Job drawing, mm, ordinate dimensions from the low corner. One solid piece. Coordinates: 2 decimals unless noted, no trailing zeros. Write each loop counter-clockwise with the first axis right and the second up, starting at its lowest first coordinate (ties: lowest second). Pieces come first, ordered by that corner, then holes. Notation, with made-up numbers: (-33.5, 3) - (-29.5, 3) arc R16 cw to (-29.5, 9) - close; hole circle Ø7 at (73, 76). An arc over 180 degrees is marked (long way). Put each result on its own line as item: value. Start each with the question number.
1. Drill centre lines: L1, parallel to X at y = 312, z = 3.75; L2, parallel to Y at x = 27, z = 2 (3 decimals). Where is each one in solid material? Low to high. Write a range as from..to.
2. Saw through at A-A, the plane z = 1.75. Write the cut outline in (x, y) (3 decimals), plus the area to 3 significant figures.
3. Drop flat-ended pins along their axis: P1, Ø3, axis at y = 66, z = 2.5, coming from the +X side; P2, Ø3, axis at y = 57, z = 4, coming from the -X side; P3, Ø3, axis at x = 395.5, z = 4.5, coming from the -Y side (3 decimals). Give the stop position or say it passes through.
4. Saw through at C-C, the plane y = 71. Write the cut outline in (x, z).
5. Saw through at B-B, the plane x = 377.5. Write the cut outline in (y, z) (3 decimals).
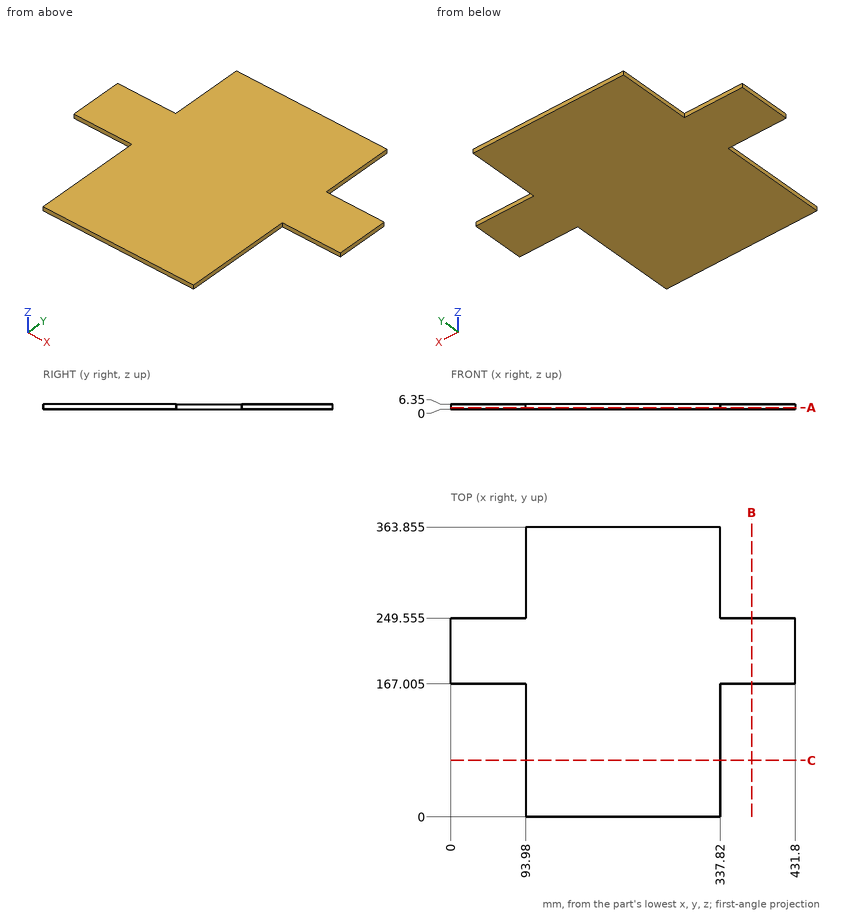
Final values:
1. L1: x = 93.98..337.82
1. L2: y = 167.005..249.555
2. outline: (0, 167.005) - (93.98, 167.005) - (93.98, 0) - (337.82, 0) - (337.82, 167.005) - (431.8, 167.005) - (431.8, 249.555) - (337.82, 249.555) - (337.82, 363.855) - (93.98, 363.855) - (93.98, 249.555) - (0, 249.555) - close
2. area: 104,000 mm²
3. P1: stops at x = 337.82
3. P2: stops at x = 93.98
3. P3: stops at y = 167.005
4. outline: (93.98, 0) - (337.82, 0) - (337.82, 6.35) - (93.98, 6.35) - close
5. outline: (167.005, 0) - (249.555, 0) - (249.555, 6.35) - (167.005, 6.35) - close
